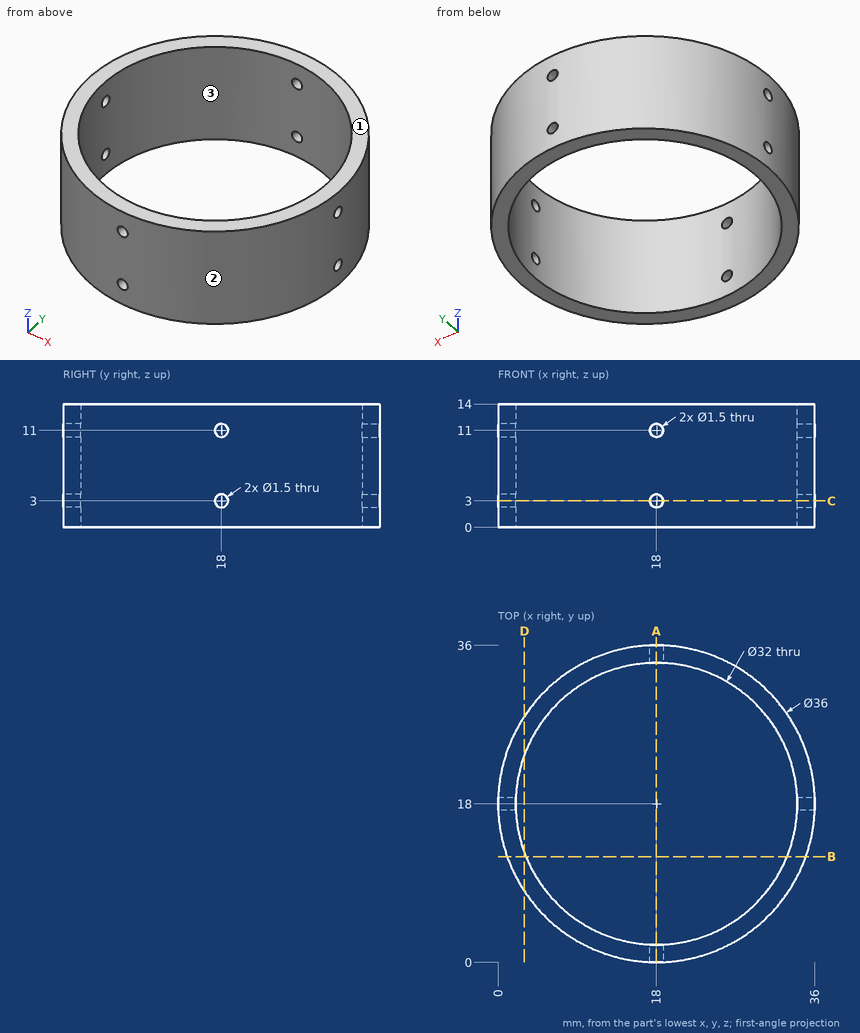
Could you check a few things on this drawing? It's one solid part, dimensions in mm from its lowest x, y, z. Coordinates: 2 decimals unless noted, no trailing zeros. Order: outer loops, then holes, each group sorted by start corner. A loop starts at its lowest first (then second) coordinate and runs counter-clockwise, first axis right, second up. Notation, with made-up numbers: M 42,-10 L 74,-10 A11 cw 74,-4 Z; hole C 69.5,3.5 d2. An arc over 180 degrees is marked long. Answer as a JSON object with one key per item and string values. Group by question number.
(1) Suppose I cut it at B-B, the plane y = 12. Please give me the cut outline in (x, z), then the cut area to 3 significant figures.
(2) For pin 1 (2.5 mm diameter, centred on y = 18, z = 3, fed in from -X); pin 2 (2 mm diameter, centred on y = 30, z = 2, fed in from -X); pin 3 (19 mm diameter, centred on x = 18, y = 18, fed in from -Z); pin 4 (3 mm diameter, centred on x = 21.5, z = 1.5, fed in from +Y), each with a flat end and sliding along its axis, tell me the tip position at first contact or that it passes through.
(3) I need wall thicknesses on probe 1 along Z at (x, y) = (18, 1.35); probe 2 along X at (y, z) = (7, 6.5); probe 3 along X at (y, z) = (17.5, 4.5). Which ranges of each line are inside material? Lowest first, please.
(4) Suppose I cut it at D-D, the plane x = 3. Please give me the cut outline in (y, z), then the cut area to 3 significant figures.
(5) Suppose I cut it at C-C, the plane z = 3. Please give me the cut outline in (x, y), then the cut area to 3 significant figures.
(6) Suppose I cut it at A-A, the plane x = 18. Please give me the cut outline in (y, z).
(7) If we mould it in two halves opening along Y, with no side actions, what happens to the marked faces 1, 2 and 3? For each: released by +Y, released by -Y, zero draft, split by the parting line, or undercut.
Values found:
{
 "1": {"outline": "M 1.03,0 L 3.17,0 L 3.17,14 L 1.03,14 Z; M 32.83,0 L 34.97,0 L 34.97,14 L 32.83,14 Z", "area": "59.9 mm^2"},
 "2": {"pin 1": "stops at x = 0", "pin 2": "stops at x = 3.75", "pin 3": "passes through", "pin 4": "stops at y = 35.89"},
 "3": {"probe 1": "z = 0 to 2.25, 3.75 to 10.25, 11.75 to 14", "probe 2": "x = 3.75 to 6.38, 29.62 to 32.25", "probe 3": "x = 0.01 to 2.01, 33.99 to 35.99"},
 "4": {"outline": "M 8.05,0 L 12.43,0 L 12.43,14 L 8.05,14 Z; M 23.57,0 L 27.95,0 L 27.95,14 L 23.57,14 Z", "area": "123 mm^2"},
 "5": {"outline": "M 0.02,17.25 A18 ccw 17.25,0.02 L 17.25,2.02 A16 cw 2.02,17.25 Z; M 0.02,18.75 L 2.02,18.75 A16 cw 17.25,33.98 L 17.25,35.98 A18 ccw Z; M 18.75,0.02 A18 ccw 35.98,17.25 L 33.98,17.25 A16 cw 18.75,2.02 Z; M 18.75,33.98 A16 cw 33.98,18.75 L 35.98,18.75 A18 ccw 18.75,35.98 Z", "area": "202 mm^2"},
 "6": {"outline": "M 0,0 L 2,0 L 2,2.25 L 0,2.25 Z; M 0,3.75 L 2,3.75 L 2,10.25 L 0,10.25 Z; M 0,11.75 L 2,11.75 L 2,14 L 0,14 Z; M 34,0 L 36,0 L 36,2.25 L 34,2.25 Z; M 34,3.75 L 36,3.75 L 36,10.25 L 34,10.25 Z; M 34,11.75 L 36,11.75 L 36,14 L 34,14 Z"},
 "7": {"face 1": "zero draft", "face 2": "split by the parting line", "face 3": "undercut"}
}
